```python
from build123d import *

# Parameters (mm, degrees)
SKETCH2_R                = 4
BOSS_EXTRUDE2_DEPTH      = 13.2
F_5_0_5_DIAMETER_HOLE1_D = 5
CHAMFER1_SIZE            = 3


with BuildPart() as part:
    # Sketch2 → Boss-Extrude2 (new body)
    with BuildSketch(Plane(origin=(0, 0, 0), x_dir=(1, 0, 0), z_dir=(0, 1, 0))):
        with BuildLine():
            Line((-14.56, -27.5), (-9.26, -27.5))
            Line((-9.26, -27.5), (-9.26, -15))
            Line((-9.26, -15), (0, -15))
            ThreePointArc((0, -15), (15, 0), (0, 15))
            Line((0, 15), (-9.26, 15))
            Line((-9.26, 15), (-9.26, 27.5))
            Line((-9.26, 27.5), (-14.56, 27.5))
            Line((-14.56, 27.5), (-14.56, -27.5))
        make_face()
        with Locations(Location((0, 0, 0), (0, 0, 270))):
            Circle(SKETCH2_R, mode=Mode.SUBTRACT)
    extrude(amount=BOSS_EXTRUDE2_DEPTH)

    # Ø5.0 (5) Diameter Hole1 (through all)
    with Locations(Plane(origin=(-9.26, 0, 0), x_dir=(0, 0, -1), z_dir=(1, 0, 0))):
        with Locations((21, 6.6), (-21, 6.6)):
            Hole(F_5_0_5_DIAMETER_HOLE1_D / 2)

    # Chamfer1
    chamfer1_edges = [part.edges().sort_by_distance(p)[0] for p in [
        (-11.91, 0, -27.5),
        (-11.91, 13.2, -27.5),
        (-11.91, 13.2, 27.5),
        (-11.91, 0, 27.5),
    ]]
    chamfer(chamfer1_edges, length=CHAMFER1_SIZE)


solid = part.part
```
Verification items for the finished model (mm, model axes). A direction names the side the tool comes from. Coordinates: 2 decimals unless noted, no trailing zeros. Write each loop counter-clockwise with the first axis right and the second up, starting at its lowest first coordinate (ties: lowest second). Pieces come first, ordered by that corner, then holes. Notation, with made-up numbers: (12, 7) - (68, 7) arc R29 ccw to (68, 39) - close; hole circle Ø5 at (65, 5.25). An arc over 180 degrees is marked (long way). One line per question, with ' | ' between items. Start each with the question number.
1. Draft check along Z on faces 4 (the cylindrical face through (-11.9, 6.7, 18.5)), 5 (the flat face through (-9.26, 5, 18.6)), 6 (the flat face through (-12, 7, 27.5)), 7 (the cylindrical face through (15, 7, 0)). Enter one of: released by +Z, released by -Z, zero draft, split by the parting line, or undercut.
2. Material ranges on line 1 along X through (y, z) = (8, 0); line 2 along Y through (x, z) = (-12.55, 21); line 3 along Z through (x, y) = (-9.5, 4.5), recorded low to high.
3. Access from +Z, -Z, +X, -X, +Y, -Y to the whole of each face (thin tool, end or side, straight path). Record for faces 1 (the cylindrical face through (-3.905, 6.508, -0.867)), 2 (the flat face through (-9.26, 7, -18)), 3 (the flat face through (-5, 7, 15)).
4. Section check C-C (y = 12.25). Enter the section's corners in (x, z).
5. Gauge pin test, flat ends, axial feed: P1, Ø3, axis at y = 2, z = 4, coming from the +X side; P2, Ø10, axis at x = -0.5, z = -16.5, coming from the -Y side; P3, Ø4.5, axis at x = -6, y = 6.5, coming from the +Z side. Record the tip position at first contact, or that the pin passes through.
6. Section check D-D (x = -10.25). Enter the section's corners in (y, z), plus the area to 3 significant figures.
7. Section check A-A (y = 6.6). Enter the section's corners in (x, z), plus the area to 3 significant figures.
8. Section check B-B (z = -21). Enter the section's corners in (x, y).
Computed values:
1) face 4: undercut | face 5: zero draft | face 6: released by +Z | face 7: split by the parting line
2) line 1: -14.56 to -4, 4 to 15 | line 2: 0 to 4.1, 9.1 to 13.2 | line 3: -27.5 to -22.36, -19.64 to 19.64, 22.36 to 27.5
3) face 1: +Y, -Y | face 2: -Z, +X, +Y, -Y | face 3: +Z, +X, +Y, -Y
4) outline: (-14.56, -25.45) - (-9.26, -25.45) - (-9.26, -15) - (0, -15) arc R15 ccw to (0, 15) - (-9.26, 15) - (-9.26, 25.45) - (-14.56, 25.45) - close; hole circle Ø8 at (0, 0)
5) P1: x = 14.79 | P2: y = 0 | P3: z = 15
6) outline: (0, -24.5) - (3, -27.5) - (10.2, -27.5) - (13.2, -24.5) - (13.2, 24.5) - (10.2, 27.5) - (3, 27.5) - (0, 24.5) - close; hole circle Ø5 at (6.6, -21); hole circle Ø5 at (6.6, 21) | area: 669 mm²
7) outline: (-14.56, -27.5) - (-9.26, -27.5) - (-9.26, -23.5) - (-14.56, -23.5) - close; (-14.56, -18.5) - (-9.26, -18.5) - (-9.26, -15) - (0, -15) arc R15 ccw to (0, 15) - (-9.26, 15) - (-9.26, 18.5) - (-14.56, 18.5) - close; (-14.56, 23.5) - (-9.26, 23.5) - (-9.26, 27.5) - (-14.56, 27.5) - close; hole circle Ø8 at (0, 0) | area: 819 mm²
8) outline: (-14.56, 0) - (-9.26, 0) - (-9.26, 4.1) - (-14.56, 4.1) - close; (-14.56, 9.1) - (-9.26, 9.1) - (-9.26, 13.2) - (-14.56, 13.2) - close
